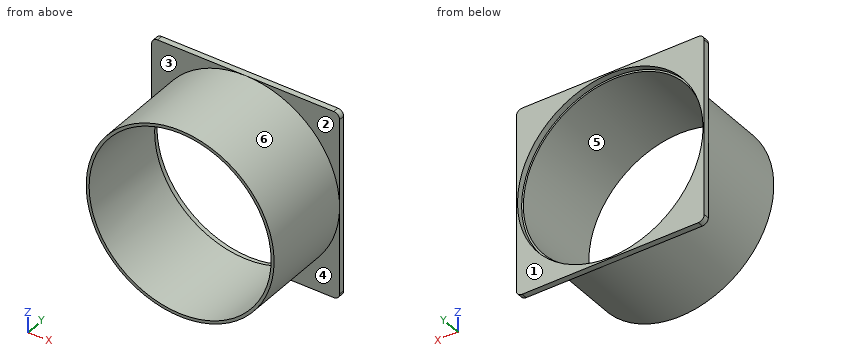
from build123d import *

# Parameters (mm, degrees)
F0_R     = 50.165
F1_DEPTH = 3.175
F2_R     = 50.8
F2_R_2   = 49.2125
F3_DEPTH = 50.8


with BuildPart() as f1:
    # F0 (on Front) → F1 (new body)
    with BuildSketch(Plane.XZ):
        with BuildLine():
            ThreePointArc((50.8, 47.625), (49.870064, 49.870064), (47.625, 50.8))
            Line((47.625, 50.8), (-47.625, 50.8))
            ThreePointArc((-47.625, 50.8), (-49.870064, 49.870064), (-50.8, 47.625))
            Line((-50.8, 47.625), (-50.8, -47.625))
            ThreePointArc((-50.8, -47.625), (-49.870064, -49.870064), (-47.625, -50.8))
            Line((-47.625, -50.8), (47.625, -50.8))
            ThreePointArc((47.625, -50.8), (49.870064, -49.870064), (50.8, -47.625))
            Line((50.8, -47.625), (50.8, 47.625))
        make_face()
        Circle(F0_R, mode=Mode.SUBTRACT)
    extrude(amount=F1_DEPTH)

    # F2 (on face) → F3 (join)
    with BuildSketch(Plane.XZ.offset(3.175)):
        Circle(F2_R)
        Circle(F2_R_2, mode=Mode.SUBTRACT)
    extrude(amount=F3_DEPTH)


solid = f1.part
CAD build for the part. Positions are in the model's coordinates, mm. Face numbers are marked on the shaded views. A direction names the side the tool comes from. Round coordinates to 2 decimals unless told otherwise and drop trailing zeros. Order: outer loops, then holes, each group sorted by start corner. A loop starts at its lowest first (then second) coordinate and runs counter-clockwise, first axis right, second up. Notation, with made-up numbers: (30, -18.5) -> (60, -18.5) arc R15 ccw to (60, 2.5) -> close; hole circle Ø4 at (60.5, 9). An arc over 180 degrees is marked (long way). Write each question's results on one line, items separated by ' | '.
1. Wall check: line 1 along Z through (x, y) = (0, -1.3) (3 decimals); line 2 along Z through (x, y) = (0, -26); line 3 along Y through (x, z) = (44.5, -36) (3 decimals). Give the ranges that are in metal, low to high. Write a range as [from, to].
Findings below:
line 1: z = [-50.8, -50.165], [50.165, 50.8] | line 2: z = [-50.8, -49.21], [49.21, 50.8] | line 3: y = [-3.175, 0]
2. Cut at C-C (y = -28.5). Give the cut face in (x, z) (1 decimal).
Findings below:
outline: circle Ø101.6 at (0, 0); hole circle Ø98.4 at (0, 0)
3. Pull direction X, two halves, no side cores. Call the marked faces 4, 5 and 6: pulls with the +X half, pulls with the -X half, needs draft (parallel to the pull), parting line crosses it, or undercut.
Findings below:
face 4: needs draft | face 5: undercut | face 6: parting line crosses it
4. 3-axis set-ups, long thin cutter, end or side, ignore diameter. For the marked faces 1, 2 and 3: which of +Z, -Z, +X, -X, +Y, -Y reach the whole face in a straight line?
Findings below:
face 1: +Z, -Z, +X, -X, +Y | face 2: +Z, +X, -Y | face 3: +Z, -X, -Y
5. Cut at A-A (z = -41.5). Give the cut face in (x, y) (3 decimals).
Findings below:
outline: (-50.8, -3.175) -> (-29.298, -3.175) -> (-29.298, -53.975) -> (-26.45, -53.975) -> (-26.45, -3.175) -> (-28.183, -3.175) -> (-28.183, 0) -> (-50.8, 0) -> close; (26.45, -53.975) -> (29.298, -53.975) -> (29.298, -3.175) -> (50.8, -3.175) -> (50.8, 0) -> (28.183, 0) -> (28.183, -3.175) -> (26.45, -3.175) -> close
6. Flat gauge pins, fed straight in: P1, Ø4, axis at y = -32.5, z = -36, coming from the -X side; P2, Ø2, axis at x = 21.5, y = -5.5, coming from the -Z side; P3, Ø3, axis at x = -25, y = -15, coming from the +Z side. Where does each tip first touch, or does it go through?
Findings below:
P1: stops at x = -37.74 | P2: stops at z = -46.48 | P3: stops at z = 45.04
7. Cut at B-B (x = 18.5). Give the cut face in (y, z) (3 decimals).
Findings below:
outline: (-53.975, -47.312) -> (-3.175, -47.312) -> (-3.175, -50.8) -> (0, -50.8) -> (0, -46.629) -> (-3.175, -46.629) -> (-3.175, -45.603) -> (-53.975, -45.603) -> close; (-53.975, 45.603) -> (-3.175, 45.603) -> (-3.175, 46.629) -> (0, 46.629) -> (0, 50.8) -> (-3.175, 50.8) -> (-3.175, 47.312) -> (-53.975, 47.312) -> close
